Autodesk Inventor part; units mm, degrees
ref_plane "YZ Plane" through (0, 0, 0) normal (1, 0, 0) x (0, 1, 0)
ref_plane "XZ Plane" through (0, 0, 0) normal (0, 1, 0) x (-1, 0, 0)
ref_plane "XY Plane" through (0, 0, 0) normal (0, 0, 1) x (1, 0, 0)
sketch "Esquisse1" plane through (0, 0, 0) normal (0, 1, 0) x (-1, 0, 0)
  line L0 (0, 0) -> (10, 0)
  line L1 (10, 0) -> (10, -10)
  line L2 (10, -10) -> (0, -10)
  line L3 (0, -10) -> (0, 0)
  dimension "d0" = 10
  dimension "d1" = 10
extrude "Extrusion1" add sketch "Esquisse1" along normal blind 40
sketch "Esquisse2" plane through (0, 0, 0) normal (1, 0, 0) x (0, 0, -1)
  line L0 (10, 0) -> (0, 0)
  line L1 (0, 0) -> (0, 40)
  point P0 (5, 35)
  dimension "d4" = 35
  dimension "d5" = 5
hole "Perçage1" at (0, 35, -5) direction (-1, 0, 0) diameter 8 depth 10 tip angle 118
sketch "Esquisse3" plane through (0, 0, 0) normal (0, -1, 0) x (1, 0, 0)
  line L0 (-10, 0) -> (0, 0)
  line L1 (-10, 0) -> (-10, -10)
  point P0 (-5, -5)
  dimension "d13" = 5
  dimension "d14" = 5
hole "Perçage2" at (-5, 0, -5) direction (0, 1, 0) diameter 4 depth 25 tip angle 118
properties part number "SupportBarreCodeuse"
Source: CAD feature listing. Evaluate the final solid. Frame: model axes, mm. Give positions to 0.01 mm unless a question says otherwise; leave off trailing zeros. Order: outer loops, then holes, each group sorted by start corner. A loop starts at its lowest first (then second) coordinate and runs counter-clockwise, first axis right, second up. Notation, with made-up numbers: (56.5, 21) -> (92.5, 21) arc R21 ccw to (92.5, 29) -> close; hole circle Ø10 at (58, 85). An arc over 180 degrees is marked (long way). Write item = value, one per line.
Item 1: Section query C-C (x = -1.25). Output: boundary loops of the cut face in (y, z), then the cut area to 3 significant figures.
Check result:
outline = (0, -10) -> (40, -10) -> (40, 0) -> (0, 0) -> close; hole circle Ø8 at (35, -5)
area = 350 mm²
Item 2: Section query D-D (y = 5). Output: boundary loops of the cut face in (x, z), then the cut area to 3 significant figures.
Check result:
outline = (-10, -10) -> (0, -10) -> (0, 0) -> (-10, 0) -> close; hole circle Ø4 at (-5, -5)
area = 87.4 mm²
Item 3: Section query A-A (y = 35). Output: boundary loops of the cut face in (x, z), then the cut area to 3 significant figures.
Check result:
outline = (-10, -10) -> (0, -10) -> (0, -9) -> (-10, -9) -> close; (-10, -1) -> (0, -1) -> (0, 0) -> (-10, 0) -> close
area = 20.0 mm²
Item 4: Section query B-B (z = -2.25). Output: boundary loops of the cut face in (x, y), then the cut area to 3 significant figures.
Check result:
outline = (-10, 0) -> (0, 0) -> (0, 32.1) -> (-10, 32.1) -> close; (-10, 37.9) -> (0, 37.9) -> (0, 40) -> (-10, 40) -> close
area = 342 mm²
Item 5: Ray query, probe 1 along Z at (x, y) = (-5, 8.5); probe 2 along Z at (x, y) = (-8, 35). Return the intervals inside material, ascending.
Check result:
probe_1 = -10 to -7, -3 to 0
probe_2 = -10 to -9, -1 to 0
Item 6: Mould query, pull axis Z, two halves, no side actions, for faces 1 (the face through (-5, 20, 0)), 2 (the face through (-5, 13, -3)), 3 (the face through (-5, 40, -5)). Classes: +Z half, -Z half, draft (parallel to the pull), parting line (faces both ways), or undercut.
Check result:
face_1 = +Z half
face_2 = undercut
face_3 = draft
